```python
from build123d import *

# Parameters (mm, degrees)
SKETCH1_R           = 0.75
SKETCH1_R_2         = 1.5
BOSS_EXTRUDE1_DEPTH = 3


with BuildPart() as part:
    # Sketch1 → Boss-Extrude1 (new body)
    with BuildSketch(Plane.XY):
        Polygon((10, 0), (10, 3), (15, 3), (15, 0), (20, 0), (20, 3), (25, 3), (25, 0), (30, 0), (30, -26), (25, -26), (25, -29), (20, -29), (20, -26), (15, -26), (15, -29), (10, -29), (10, -26), (5, -26), (5, -29), (0, -29), (0, -26), (-18.49, -26), (-18.49, 0), (0, 0), align=None)
        with Locations((20.5, -5.5)):
            Circle(SKETCH1_R, mode=Mode.SUBTRACT)
        with Locations((26.995190528, -9.25)):
            Circle(SKETCH1_R, mode=Mode.SUBTRACT)
        with Locations((26.995190528, -16.75)):
            Circle(SKETCH1_R, mode=Mode.SUBTRACT)
        with Locations((20.5, -20.5)):
            Circle(SKETCH1_R, mode=Mode.SUBTRACT)
        with Locations((14.004809472, -16.75)):
            Circle(SKETCH1_R, mode=Mode.SUBTRACT)
        with Locations((14.004809472, -9.25)):
            Circle(SKETCH1_R, mode=Mode.SUBTRACT)
        with Locations((20.5, -13)):
            Circle(SKETCH1_R_2, mode=Mode.SUBTRACT)
    extrude(amount=BOSS_EXTRUDE1_DEPTH)


solid = part.part
```
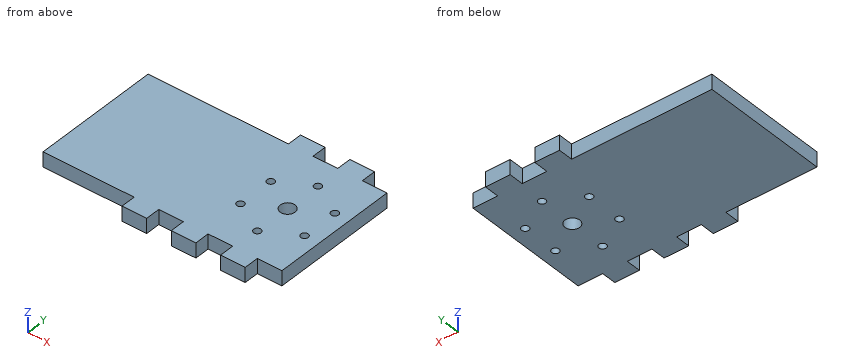
Geometry: final body of the model. Coordinates: model frame, mm. Round coordinates to 2 decimals unless told otherwise and drop trailing zeros. Write each loop counter-clockwise with the first axis right and the second up, starting at its lowest first coordinate (ties: lowest second). Pieces come first, ordered by that corner, then holes.
Item 1: Pin query (flat end, axial travel): P1, Ø0.9, axis at x = -5.5, z = 2, coming from the +Y side; P2, Ø0.9, axis at y = 2, z = 2, coming from the +X side; P3, Ø1.5, axis at x = 28, z = 1.5, coming from the -Y side. Return the tip coordinate at first contact, or that it passes through.
Item 2: Section query C-C (z = 0.7). Give the number of separate pieces and of enclosed holes in the cut face, plus the area to 3 significant figures.
Item 3: Section query D-D (y = -16.75). Return loops of the section in (x, z).
Item 4: Section query A-A (y = -13). Return loops of the section in (x, z), plus the area to 3 significant figures.
Item 5: Material intervals for L1, parallel to Y at x = 20.5, z = 1.8; L2, parallel to Y at x = 27, z = 1.45; L3, parallel to X at y = -9, z = 1.3, sorted ascending.
Item 6: Section query B-B (x = 20.5). Return loops of the section in (y, z).
Completed:
1. P1: stops at y = 0
1. P2: stops at x = 25
1. P3: stops at y = -26
2. separate pieces: 1
2. enclosed holes: 7
2. area: 1,320 mm2
3. outline: (-18.49, 0) - (13.25, 0) - (13.25, 3) - (-18.49, 3) - close; (14.75, 0) - (26.25, 0) - (26.25, 3) - (14.75, 3) - close; (27.75, 0) - (30, 0) - (30, 3) - (27.75, 3) - close
4. outline: (-18.49, 0) - (19, 0) - (19, 3) - (-18.49, 3) - close; (22, 0) - (30, 0) - (30, 3) - (22, 3) - close
4. area: 136 mm2
5. L1: y = -29 to -21.25, -19.75 to -14.5, -11.5 to -6.25, -4.75 to 3
5. L2: y = -26 to -17.5, -16 to -10, -8.5 to 0
5. L3: x = -18.49 to 13.3, 14.71 to 26.29, 27.7 to 30
6. outline: (-29, 0) - (-21.25, 0) - (-21.25, 3) - (-29, 3) - close; (-19.75, 0) - (-14.5, 0) - (-14.5, 3) - (-19.75, 3) - close; (-11.5, 0) - (-6.25, 0) - (-6.25, 3) - (-11.5, 3) - close; (-4.75, 0) - (3, 0) - (3, 3) - (-4.75, 3) - close
